The model under review builds one solid part; all positions refer to its coordinate system, in mm. Face numbers are marked on the shaded views. A direction names the side the tool comes from. Round coordinates to 2 decimals unless told otherwise and drop trailing zeros. Loops run counter-clockwise (first coordinate to the right, second up) from the corner with the lowest first, then second, coordinate; pieces in that order, holes last. Notation, with made-up numbers: (50.25, 61.25) -> (54.25, 61.25) arc R23 cw to (54.25, 95.25) -> close; hole circle Ø1 at (-19, 65.25). An arc over 180 degrees is marked (long way). Return JSON: item names as keys, results as strings. Group by question number.
Autodesk Inventor part; units mm, degrees
ref_plane "YZ Plane" through (0, 0, 0) normal (1, 0, 0) x (0, 1, 0)
ref_plane "XZ Plane" through (0, 0, 0) normal (0, 1, 0) x (-1, 0, 0)
ref_plane "XY Plane" through (0, 0, 0) normal (0, 0, 1) x (1, 0, 0)
sketch "スケッチ1" plane through (0, 0, 0) normal (1, 0, 0) x (0, 1, 0)
  line L0 (45, 0) -> (0, 0)
  line L1 (0, 0) -> (0, -11.5)
  line L2 (0, -11.5) -> (45, -11.5)
  line L3 (45, -11.5) -> (45, 0)
  dimension "d0" = 45
  dimension "d1" = 11.5
extrude "押し出し1" add sketch "スケッチ1" along normal blind 2
sketch "スケッチ2" plane through (2, 0, 0) normal (1, 0, 0) x (0, 0, -1)
  circle A0 centre (1.5, 43) radius 0.8
  circle A1 centre (9.4807, 43) radius 0.8
  circle A2 centre (9.5, 2) radius 0.8
  circle A3 centre (1.5, 2) radius 0.8
  circle A4 centre (5.5, 22.5) radius 0.8
  point P0 (0, 0)
extrude "押し出し2" cut sketch "スケッチ2" against normal through all
fillet "フィレット1" radius 2 2 edges at (1, 45, -11.5) (1, 0, -11.5)
sketch "スケッチ3" plane through (0, 0, 0) normal (-1, 0, 0) x (0, 0, 1)
  circle A0 centre (-5.5, 22.5) radius 0.8
  circle A1 centre (-5.5, 22.5) radius 10
  line L0 (-2, 45) -> (0, 45)
  line L1 (0, 45) -> (0, 0)
  line L2 (0, 0) -> (-2, 0)
  line L3 (-2, 0) -> (-2, 45)
  line L4 (-9.5, 45) -> (0, 45)
  line L5 (0, 0) -> (-9.5, 0)
  circle A2 centre (-5.5, 22.5) radius 0.8
  arc A3 (-11.5, 2) -> (-9.5, 0) centre (-9.5, 2) ccw
  line L6 (0, 0) -> (-9.5, 0)
  line L7 (0, 45) -> (0, 0)
  line L8 (-9.5, 45) -> (0, 45)
  arc A4 (-9.5, 45) -> (-11.5, 43) centre (-9.5, 43) ccw
  line L9 (-11.5, 2) -> (-11.5, 43)
  circle A5 centre (-1.5, 43) radius 0.8
  circle A6 centre (-1.5, 2) radius 0.8
  point P0 (-2, 31.8675)
  point P1 (-2, 13.1325)
  point P2 (0, 14.1484)
  point P3 (0, 30.8516)
  point P4 (-11.5, 14.5)
  point P5 (-11.5, 30.5)
  point P6 (-2, 45)
  point P7 (-2, 43.6245)
  point P8 (-2, 42.3755)
  point P9 (-2, 2.6245)
  point P10 (-2, 1.3755)
  dimension "d7" = 20
  dimension "d34" = 2
extrude "押し出し3" add sketch "スケッチ3" against normal blind 35 contours A1 L3 A5 L0 L1 | L1 L2 L3 A6 A1
sketch "スケッチ6" plane through (0, 0, 0) normal (0, 0, 1) x (1, 0, 0)
  line L0 (5, 37.5) -> (30, 37.5) construction
  line L1 (30, 37.5) -> (30, 7.5) construction
  line L2 (30, 7.5) -> (5, 7.5) construction
  line L3 (5, 7.5) -> (5, 37.5) construction
  line L4 (0, 45) -> (35, 45)
  line L5 (0, 0) -> (35, 0)
  line L6 (35, 45) -> (35, 30.8516)
  line L7 (0, 45) -> (0, 0)
  circle A0 centre (5, 37.5) radius 0.8
  circle A1 centre (30, 37.5) radius 0.8
  circle A2 centre (5, 7.5) radius 0.8
  circle A3 centre (30, 7.5) radius 0.8
  dimension "d35" = 25
  dimension "d36" = 30
  dimension "d37" = 7.5
  dimension "d38" = 7.5
  dimension "d39" = 5
  dimension "d40" = 5
  dimension "d41" = 1.6
  dimension "d42" = 1.6
  dimension "d43" = 1.6
  dimension "d44" = 1.6
extrude "押し出し6" cut sketch "スケッチ6" against normal through all
equation "\"d37\" = d38"
equation "\"d39\" = d40"
properties part number "bluetooth_setter"
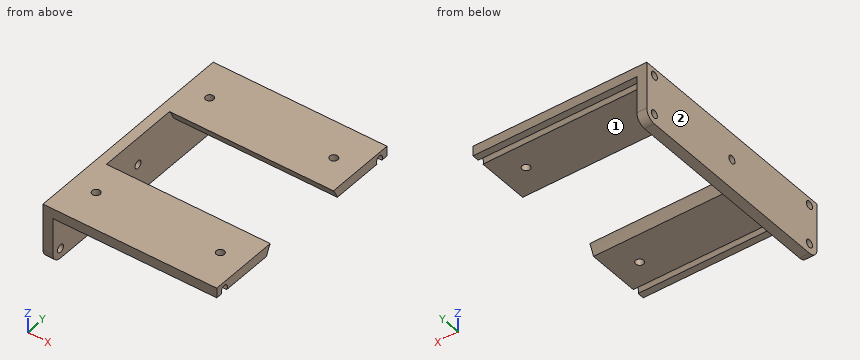
1. Wall thickness on line 1 (Z direction, x = 1.1, y = 43); line 2 (Y direction, x = 30, z = -1.05); line 3 (Y direction, x = 5, z = -1.4): over which ranges is each line inside the solid? List them lowest first.
2. We need section D-D, the plane y = 22.5. Write out the cut boundary in (x, z), then the cut area to 3 significant figures.
3. We need section A-A, the plane y = 37.5. Write out the cut boundary in (x, z).
4. We need section C-C, the plane z = -1.5. Write out the cut boundary in (x, y).
5. For P1, Ø1, axis at y = 2, z = -9.5, coming from the -X side; P2, Ø2, axis at x = 11.5, y = 10.5, coming from the -Z side; P3, Ø1.5, axis at y = 31, z = -5, coming from the +X side, all flat-tipped, find the tip position at first contact; note any pin that passes through.
6. We need section B-B, the plane x = 26. Write out the cut boundary in (y, z), then the cut area to 3 significant figures.
7. Tool access review of the marked faces 1 and 2: name each direction out of +Z, -Z, +X, -X, +Y, -Y from which nothing blocks a thin tool from reaching the whole face with its end or side.
Check sheet entries:
{
 "1": {"line 1": "z = -11.5 to -10.28, -8.68 to -2.3, -0.7 to 0", "line 2": "y = 0 to 1.34, 2.66 to 6.7, 8.3 to 13.54, 31.46 to 36.7, 38.3 to 42.34, 43.66 to 45", "line 3": "y = 0 to 1.21, 2.79 to 6.7, 8.3 to 13.38, 31.62 to 36.7, 38.3 to 42.21, 43.79 to 45"},
 "2": {"outline": "(0, -11.5) -> (2, -11.5) -> (2, -6.3) -> (0, -6.3) -> close; (0, -4.7) -> (2, -4.7) -> (2, 0) -> (0, 0) -> close", "area": "19.8 mm²"},
 "3": {"outline": "(0, -11.5) -> (2, -11.5) -> (2, -2) -> (4.2, -2) -> (4.2, 0) -> (0, 0) -> close; (5.8, -2) -> (29.2, -2) -> (29.2, 0) -> (5.8, 0) -> close; (30.8, -2) -> (35, -2) -> (35, 0) -> (30.8, 0) -> close"},
 "4": {"outline": "(0, 0) -> (35, 0) -> (35, 1.2) -> (0, 1.2) -> close; (0, 2.8) -> (35, 2.8) -> (35, 13.33) -> (2, 13.33) -> (2, 31.67) -> (35, 31.67) -> (35, 42.2) -> (0, 42.2) -> close; (0, 43.8) -> (35, 43.8) -> (35, 45) -> (0, 45) -> close; hole circle Ø1.6 at (5, 7.5); hole circle Ø1.6 at (5, 37.5); hole circle Ø1.6 at (30, 7.5); hole circle Ø1.6 at (30, 37.5)"},
 "5": {"P1": "passes through", "P2": "stops at z = -2", "P3": "stops at x = 2"},
 "6": {"outline": "(0, -2) -> (1.38, -2) arc R0.8 cw (long way) to (2.62, -2) -> (13.13, -2) arc R10 cw to (14.15, 0) -> (0, 0) -> close; (30.85, 0) arc R10 cw to (31.87, -2) -> (42.38, -2) arc R0.8 cw (long way) to (43.62, -2) -> (45, -2) -> (45, 0) -> close", "area": "50.9 mm²"},
 "7": {"face 1": "-Z, +X, +Y, -Y", "face 2": "+Z, -Z, -X, +Y, -Y"}
}
